Could you check a few things on this drawing? It's one solid part, dimensions in mm from its lowest x, y, z. A direction names the side the tool comes from. Coordinates: 2 decimals unless noted, no trailing zeros. Loops run counter-clockwise (first coordinate to the right, second up) from the corner with the lowest first, then second, coordinate; pieces in that order, holes last.
1) For the marked faces 4, 5 and 6, which set-ups out of +Z, -Z, +X, -X, +Y, -Y let a thin tool reach every point of the face, with its end or its side?
2) Will these pins go through, and if not, where does the flat tip stop? P1, Ø1.5, axis at y = 23, z = 7, coming from the -X side; P2, Ø1, axis at y = 10, z = 3, coming from the -X side; P3, Ø8, axis at x = 5, y = 23, coming from the -Z side; P4, Ø6.5, axis at x = 10, y = 8.5, coming from the +Z side.
3) Imagine slicing it at D-D on z = 6. Please give me the cut outline in (x, y).
4) If I drill on line 1 along Y through (x, z) = (13.5, 3.2); line 2 along Z through (x, y) = (16.5, 8), over which ranges is the centre line in solid material (lowest first)?
5) Imagine slicing it at B-B on x = 13.5. Please give me the cut outline in (y, z), plus the area to 3 significant figures.
6) Thinking about a two-plate mould opening in Y: for the marked faces 1, 2 and 3, which applies, released by +Y, released by -Y, zero draft, split by the parting line, or undercut?
7) Imagine slicing it at A-A on z = 2.25. Please give me the cut outline in (x, y), plus the area to 3 significant figures.
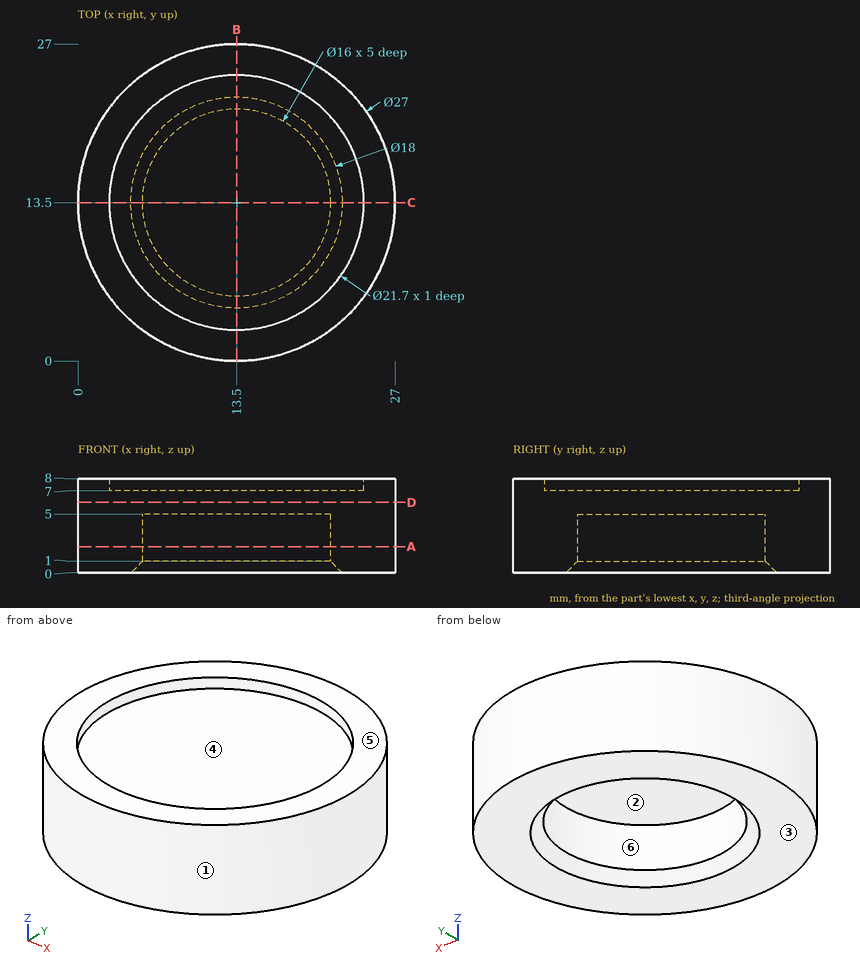
Filled in:
1. face 4: +Z
1. face 5: +Z, +X, -X, +Y, -Y
1. face 6: -Z
2. P1: stops at x = 3.22
2. P2: stops at x = 0.34
2. P3: stops at z = 0
2. P4: stops at z = 7
3. outline: circle Ø27 at (13.5, 13.5)
4. line 1: y = 0 to 5.5, 21.5 to 27
4. line 2: z = 5 to 7
5. outline: (0, 0) - (4.5, 0) - (5.5, 1) - (5.5, 5) - (21.5, 5) - (21.5, 1) - (22.5, 0) - (27, 0) - (27, 8) - (24.35, 8) - (24.35, 7) - (2.65, 7) - (2.65, 8) - (0, 8) - close
5. area: 113 mm2
6. face 1: split by the parting line
6. face 2: undercut
6. face 3: zero draft
7. outline: circle Ø27 at (13.5, 13.5); hole circle Ø16 at (13.5, 13.5)
7. area: 371 mm2
